from build123d import *

# Parameters (mm, degrees)
EXTRUDE_THIN1_DEPTH = 508
FILLET1_R           = 1.27


with BuildPart() as part:
    # Sketch1 → Extrude-Thin1 (new body)
    with BuildSketch(Plane.XY):
        with BuildLine():
            Line((0, 9.525), (0, 6.35))
            Line((0, 6.35), (-18.25625, 6.35))
            ThreePointArc((-18.25625, 6.35), (-22.746378061, 4.490128061), (-24.60625, 0))
            Line((-24.60625, 0), (-31.75, 0))
            Line((-31.75, 0), (-31.75, 20.6375))
            Line((-31.75, 20.6375), (-35.71875, 20.6375))
            Line((-35.71875, 20.6375), (-35.71875, 25.4))
            ThreePointArc((-35.71875, 25.4), (-39.20672008, 26.631209101), (-41.148892003, 29.779189303))
            Line((-41.148892003, 29.779189303), (-44.099857997, 43.392900498))
            ThreePointArc((-44.099857997, 43.392900498), (-46.562785495, 46.913451124), (-50.8, 47.625))
            Line((-50.8, 47.625), (-50.8, 54.61))
            ThreePointArc((-50.8, 54.61), (-49.566819219, 56.788032031), (-47.064705882, 56.851176471))
            Line((-47.064705882, 56.851176471), (-42.8625, 54.61))
            Line((-42.8625, 54.61), (-43.460147059, 53.489411765))
            Line((-43.460147059, 53.489411765), (-47.662352941, 55.730588235))
            ThreePointArc((-47.662352941, 55.730588235), (-48.913409609, 55.699016016), (-49.53, 54.61))
            Line((-49.53, 54.61), (-49.53, 49.042089801))
            ThreePointArc((-49.53, 49.042089801), (-45.244779615, 47.529461477), (-42.858682681, 43.661942943))
            Line((-42.858682681, 43.661942943), (-39.907716688, 30.048231748))
            ThreePointArc((-39.907716688, 30.048231748), (-37.879157823, 27.254280646), (-34.44875, 26.862469466))
            Line((-34.44875, 26.862469466), (-34.44875, 21.9075))
            Line((-34.44875, 21.9075), (-30.48, 21.9075))
            Line((-30.48, 21.9075), (-30.48, 1.27))
            Line((-30.48, 1.27), (-25.769671325, 1.27))
            ThreePointArc((-25.769671325, 1.27), (-23.17493885, 5.819871133), (-18.25625, 7.62))
            Line((-18.25625, 7.62), (-1.27, 7.62))
            Line((-1.27, 7.62), (-1.27, 9.525))
            Line((-1.27, 9.525), (0, 9.525))
        make_face()
    extrude(amount=-EXTRUDE_THIN1_DEPTH)

    # Fillet1
    fillet1_edges = [part.edges().sort_by_distance(p)[0] for p in [
        (-34.44875, 26.862469466, -254),
        (-30.48, 21.9075, -254),
        (0, 6.35, -254),
        (-24.60625, 0, -254),
        (-31.75, 0, -254),
        (-35.71875, 20.6375, -254),
        (-50.8, 47.625, -254),
    ]]
    fillet(fillet1_edges, radius=FILLET1_R)


solid = part.part
Geometry: final body of the model. Coordinates: model frame, mm. A direction names the side the tool comes from. Round coordinates to 2 decimals unless told otherwise and drop trailing zeros. Write each loop counter-clockwise with the first axis right and the second up, starting at its lowest first coordinate (ties: lowest second). Pieces come first, ordered by that corner, then holes. Notation, with made-up numbers: M 88.5,63.5 L 146.5,63.5 A25 cw 146.5,88.5 Z; hole C 8,-20.5 d6. An arc over 180 degrees is marked long. Write item = value, one per line.
Item 1: Pull-direction query (X, two-part tool) for faces 1 (the face through (-10, 7.62, -250)), 2 (the face through (-31, 20, -508)), 3 (the face through (-42.604, 36.491, -250.444)), 4 (the face through (-30.48, 11, -250)); classes: pulls with the +X half, pulls with the -X half, needs draft (parallel to the pull), parting line crosses it, or undercut.
Findings:
face_1 = undercut
face_2 = needs draft
face_3 = pulls with the -X half
face_4 = undercut
Item 2: Access query for faces 5 (the face through (-31.75, 11, -250)), 6 (the face through (-31, 20, 0)), 7 (the face through (-10, 6.35, -250)). Directions: +Z, -Z, +X, -X, +Y, -Y. A direction counts if a zero-diameter tool reaches every point of the face in a straight line with its end or side. Return the directions, or none.
Findings:
face_5 = +Z, -Z, -X, -Y
face_6 = +Z, +X, -X, +Y, -Y
face_7 = +Z, -Z, +X, -Y
Item 3: Pin query (flat end, axial travel): P1, Ø12, axis at y = 45, z = -212, coming from the +X side; P2, Ø1, axis at x = -0.5, z = -133.5, coming from the +Y side (3 decimals); P3, Ø4, axis at y = 23, z = -281, coming from the -X side; P4, Ø8, axis at x = -38.5, y = 11, coming from the -Z side. Return the tip coordinate at first contact, or that it passes through.
Findings:
P1 = -41.85
P2 = 9.525
P3 = -35.72
P4 = through
Item 4: Section query B-B on x = -7.5. Return loops of the section in (y, z).
Findings:
outline = M 6.35,-508 L 7.62,-508 L 7.62,0 L 6.35,0 Z
Item 5: Section query A-A on y = 16. Return loops of the section in (x, z).
Findings:
outline = M -31.75,-508 L -30.48,-508 L -30.48,0 L -31.75,0 Z
Item 6: Material intervals for line 1 along Y through (x, z) = (-4.5, -131.5); line 2 along X through (y, z) = (14.5, -317.5); line 3 along Y through (x, z) = (-32, -360), sorted ascending. Write a range as [from, to].
Findings:
line_1 = [6.35, 7.62]
line_2 = [-31.75, -30.48]
line_3 = [20.64, 21.91]
